```python
from build123d import *

# Parameters (mm, degrees)
SKETCH1_R           = 330
SKETCH1_R_2         = 247.5
BOSS_EXTRUDE1_DEPTH = 70
SKETCH2_R           = 28.575
CUT_EXTRUDE1_DEPTH  = 131


with BuildPart() as part:
    # Sketch1 → Boss-Extrude1 (new body)
    with BuildSketch(Plane.XY):
        Circle(SKETCH1_R)
        Circle(SKETCH1_R_2, mode=Mode.SUBTRACT)
        Circle(SKETCH1_R_2)
    extrude(amount=BOSS_EXTRUDE1_DEPTH)

    # Sketch2 → Cut-Extrude1 (cut)
    with BuildSketch(Plane.XY):
        with Locations((0, 290)):
            Circle(SKETCH2_R)
        with Locations((145, 251.147367097)):
            Circle(SKETCH2_R)
        with Locations((251.147367097, 145)):
            Circle(SKETCH2_R)
        with Locations((290, 0)):
            Circle(SKETCH2_R)
        with Locations((251.147367098, -145)):
            Circle(SKETCH2_R)
        with Locations((145, -251.147367097)):
            Circle(SKETCH2_R)
        with Locations((0, -290)):
            Circle(SKETCH2_R)
        with Locations((-145, -251.147367097)):
            Circle(SKETCH2_R)
        with Locations((-251.147367097, -145)):
            Circle(SKETCH2_R)
        with Locations((-290, 0)):
            Circle(SKETCH2_R)
        with Locations((-251.147367097, 145)):
            Circle(SKETCH2_R)
        with Locations((-145, 251.147367097)):
            Circle(SKETCH2_R)
    extrude(amount=CUT_EXTRUDE1_DEPTH, mode=Mode.SUBTRACT)


solid = part.part
```
The model under review builds one solid part; all positions refer to its coordinate system, in mm. Give positions to 0.01 mm unless a question says otherwise; leave off trailing zeros. Write each loop counter-clockwise with the first axis right and the second up, starting at its lowest first coordinate (ties: lowest second). Pieces come first, ordered by that corner, then holes. Notation, with made-up numbers: (58.25, -34) - (97.25, -34) arc R17 cw to (97.25, -29) - close; hole circle Ø10 at (-1, 33). An arc over 180 degrees is marked (long way). Answer in a Markdown table with one row per item. Add a question column.
1. We need section D-D on y = 270.5. Write out the cut boundary in (x, z), then the cut area to 3 significant figures.
2. Draft analysis for pull direction X (two halves, no side actions). For faces 1 (the cylindrical face through (-3.72, -261.67, 34.51)), 2 (the cylindrical face through (-71.538, -322.153, 34.51)), 3 (the flat face through (-5, 5, 70)), state which applies: +X half, -X half, draft (parallel to the pull), parting line (faces both ways), or undercut.
3. We need section C-C on x = 290. Write out the cut boundary in (y, z) (3 decimals), then the cut area to 3 significant figures.
4. Insertion check: P1, Ø1, axis at y = -228, z = 36, coming from the -X side; P2, Ø12, axis at x = -139, z = 10.5, coming from the +Y side; P3, Ø1, axis at y = -50, z = 37, coming from the +X side. Each pin has a flat end and moves straight along its axis. Give the tip position at first contact, or say it passes through.
5. We need section A-A on x = 0. Write out the cut boundary in (y, z) (3 decimals).
6. Wall thickness on line 1 along X through (y, z) = (4.5, 48.5); line 2 along Y through (x, z) = (0, 38) (3 decimals); line 3 along Y through (x, z) = (7, 49): over which ranges is each line inside the solid? List them lowest first. Write a range as [from, to].
Ans:
| question | item | result |
|---|---|---|
| 1 | outline | (-189.02, 0) - (-166.02, 0) - (-166.02, 70) - (-189.02, 70) - close; (-123.98, 0) - (-20.89, 0) - (-20.89, 70) - (-123.98, 70) - close; (20.89, 0) - (123.98, 0) - (123.98, 70) - (20.89, 70) - close; (166.02, 0) - (189.02, 0) - (189.02, 70) - (166.02, 70) - close |
| 1 | area | 17,700 mm^2 |
| 2 | face 1 | undercut |
| 2 | face 2 | parting line |
| 2 | face 3 | draft |
| 3 | outline | (-157.48, 0) - (-28.575, 0) - (-28.575, 70) - (-157.48, 70) - close; (28.575, 0) - (157.48, 0) - (157.48, 70) - (28.575, 70) - close |
| 3 | area | 18,000 mm^2 |
| 4 | P1 | stops at x = -239.05 |
| 4 | P2 | stops at y = 302.01 |
| 4 | P3 | stops at x = 326.27 |
| 5 | outline | (-330, 0) - (-318.575, 0) - (-318.575, 70) - (-330, 70) - close; (-261.425, 0) - (261.425, 0) - (261.425, 70) - (-261.425, 70) - close; (318.575, 0) - (330, 0) - (330, 70) - (318.575, 70) - close |
| 6 | line 1 | x = [-329.97, -318.22], [-261.78, 261.78], [318.22, 329.97] |
| 6 | line 2 | y = [-330, -318.575], [-261.425, 261.425], [318.575, 330] |
| 6 | line 3 | y = [-329.93, -317.7], [-262.3, 262.3], [317.7, 329.93] |
